from build123d import *

# Parameters (mm, degrees)
CHAMFER1_SIZE = 10


with BuildPart() as part:
    # Sketch1 → Revolve1 (revolve)
    with BuildSketch(Plane.XY, mode=Mode.PRIVATE) as revolve1_sk:
        Polygon((36.25, 0), (36.25, 10), (47, 10), (47, 35), (57, 35), (57, 0), align=None)
    revolve(revolve1_sk.sketch.rotate(Axis((0, 630.278330928, 0), (0, -1, 0)), 90), axis=Axis((0, 630.278330928, 0), (0, -1, 0)))

    # Chamfer1
    chamfer1_edges = [part.edges().sort_by_distance(p)[0] for p in [
        (0, 35, -57),
    ]]
    chamfer(chamfer1_edges, length=CHAMFER1_SIZE - 0.0001)  # a hair under: the kernel refuses the full size


solid = part.part
Design review of the part built by this model. Coordinates are the model's own, in mm. Round coordinates to 2 decimals unless told otherwise and drop trailing zeros. Write each loop counter-clockwise with the first axis right and the second up, starting at its lowest first coordinate (ties: lowest second). Pieces come first, ordered by that corner, then holes.
Item 1: Draft analysis for pull direction Z (two halves, no side actions). For faces 1 (the cylindrical face through (-46.6, 22.68, -6.12)), 2 (the cylindrical face through (32.16, 5.07, 16.73)), 3 (the flat face through (37, 0, -1)), 4 (the cylindrical face through (50.57, 12.33, 26.3)), state which applies: released by +Z, released by -Z, zero draft, split by the parting line, or undercut.
Item 2: Consider section C-C on y = 17. Give the boundary of the cut face in (x, z).
Item 3: Wall thickness on L1, parallel to Y at x = -11, z = 43; L2, parallel to Z at x = 42.5, y = 12.5; L3, parallel to Z at x = -14, y = 30: over which ranges is each line inside the solid? List them lowest first.
Item 4: For pin 1 Ø2 at (y, z) = (31, 22.5) entering from +X; pin 2 Ø12 at (x, y) = (16, 3.5) entering from -Z; pin 3 Ø4 at (x, y) = (19, 7.5) entering from -Z, all flat-tipped, find the tip position at first contact; note any pin that passes through.
Item 5: Consider section D-D on y = 29.5. Give the boundary of the cut face in (x, z), and give its area (3 significant figures).
Check values:
1. face 1: undercut
1. face 2: undercut
1. face 3: zero draft
1. face 4: split by the parting line
2. outline: circle Ø114 at (0, 0); hole circle Ø94 at (0, 0)
3. L1: y = 0 to 10
3. L2: z = -37.98 to -20.07, 20.07 to 37.98
3. L3: z = -50.08 to -44.87, 44.87 to 50.08
4. pin 1: stops at x = 46.98
4. pin 2: stops at z = -56.12
4. pin 3: stops at z = -54.41
5. outline: circle Ø105 at (0, 0); hole circle Ø94 at (0, 0)
5. area: 1,720 mm2
